Autodesk Inventor part; units mm, degrees
ref_plane "YZ Plane" through (0, 0, 0) normal (1, 0, 0) x (0, 1, 0)
ref_plane "XZ Plane" through (0, 0, 0) normal (0, 1, 0) x (-1, 0, 0)
ref_plane "XY Plane" through (0, 0, 0) normal (0, 0, 1) x (1, 0, 0)
sketch "Sketch1" plane through (0, 0, 0) normal (0, 0, 1) x (1, 0, 0)
  line L0 (0, 0) -> (20, 0)
  line L1 (20, 0) -> (20, 25)
  line L2 (20, 25) -> (0, 25)
  line L3 (0, 25) -> (0, 0)
  line L4 (5, 16.5) -> (17, 16.5)
  line L5 (17, 16.5) -> (17, 8.5)
  line L6 (17, 8.5) -> (5, 8.5)
  line L7 (5, 8.5) -> (5, 16.5)
  point P0 (17, 12.5)
  point P1 (20, 12.5)
  dimension "d0" = 20
  dimension "d2" = 25
  dimension "d3" = 8
  dimension "d4" = 12
  dimension "d5" = 3
extrude "Extrusion1" add sketch "Sketch1" along normal blind 3
sketch "Sketch2" plane through (0, 0, 3) normal (0, 0, 1) x (1, 0, 0)
  line L0 (17, 16.5) -> (17, 8.5)
  line L1 (17, 8.5) -> (5, 8.5)
  line L2 (5, 8.5) -> (5, 16.5)
  line L3 (5, 16.5) -> (17, 16.5)
  line L4 (20, 0) -> (20, 25)
  line L5 (20, 19.5) -> (20, 5.5)
  line L6 (20, 5.5) -> (2, 5.5)
  line L7 (2, 5.5) -> (2, 19.5)
  line L8 (2, 19.5) -> (20, 19.5)
extrude "Extrusion2" add sketch "Sketch2" along normal blind 7
sketch "Sketch3" plane through (0, 0, 10) normal (0, 0, 1) x (1, 0, 0)
  line L0 (17, 8.5) -> (5, 8.5)
  line L1 (5, 8.5) -> (5, 16.5)
  line L2 (5, 16.5) -> (17, 16.5)
  line L3 (17, 16.5) -> (17, 8.5)
  point P0 (0, 0)
extrude "Extrusion3" add sketch "Sketch3" against normal blind 3
sketch "Sketch4" plane through (0, 0, 0) normal (0, 0, -1) x (-1, 0, 0)
  line L0 (0, 0) -> (-20, 0)
  line L1 (-20, 25) -> (0, 25)
  line L2 (-20, 0) -> (-20, 25)
  circle A0 centre (-16.75, 22) radius 1.25
  circle A1 centre (-12.25, 22) radius 1.25
  circle A2 centre (-7.75, 22) radius 1.25
  circle A3 centre (-3.25, 22) radius 1.25
  circle A4 centre (-16.75, 3) radius 1.25
  circle A5 centre (-12.25, 3) radius 1.25
  circle A6 centre (-7.75, 3) radius 1.25
  circle A7 centre (-3.25, 3) radius 1.25
  line L3 (-12.25, 22) -> (-7.75, 22)
  line L4 (-17, 8.5) -> (-17, 16.5)
  line L5 (-17, 16.5) -> (-5, 16.5)
  circle A8 centre (-9, 12.5) radius 1.6
  line L6 (-5, 16.5) -> (-5, 8.5)
  point P0 (-10, 22)
  point P1 (-10, 25)
  point P2 (-17, 12.5)
  point P3 (-11, 16.5)
  dimension "d12" = 2.5
  dimension "d13" = 2.5
  dimension "d14" = 2.5
  dimension "d15" = 2.5
  dimension "d16" = 2.5
  dimension "d17" = 2.5
  dimension "d18" = 2.5
  dimension "d19" = 2.5
  dimension "d20" = 4.5
  dimension "d21" = 4.5
  dimension "d22" = 4.5
  dimension "d23" = 3
  dimension "d24" = 3
  dimension "d27" = 3.2
  dimension "d28" = 4
extrude "Extrusion4" cut sketch "Sketch4" against normal blind 10
equation "\"d21\" = d20"
equation "\"d22\" = d20"
equation "\"d24\" = d23"
properties part number "end limit holder"
Can you work these out from the model? Positions are in its coordinate system, mm. A direction names the side the tool comes from. Coordinates: 2 decimals unless noted, no trailing zeros. Loops run counter-clockwise (first coordinate to the right, second up) from the corner with the lowest first, then second, coordinate; pieces in that order, holes last.
1) Imagine slicing it at D-D on y = 12.5. List the corners of the cut face in (x, z) for me, plus the area to 3 significant figures.
2) For pin 1 (4 mm diameter, centred on x = 16.75, y = 3, fed in from -Z); pin 2 (3 mm diameter, centred on x = 7.75, y = 22, fed in from +Z); pin 3 (2 mm diameter, centred on x = 3.25, y = 3, fed in from +Z); pin 4 (4 mm diameter, centred on x = 8.5, y = 13.5, fed in from -Z), each with a flat end and sliding along its axis, tell me the tip position at first contact or that it passes through.
3) Imagine slicing it at C-C on z = 8.5. List the corners of the cut face in (x, y) for me.
4) Imagine slicing it at A-A on y = 21.25. List the corners of the cut face in (x, z) for me.
5) Imagine slicing it at B-B on x = 12.25. List the corners of the cut face in (y, z) for me, plus the area to 3 significant figures.
6) Thinking about a two-plate mould opening in X: for faces 4 (the flat face through (2, 12, 6)), 5 (the flat face through (5, 12, 3)), 6 (the flat face through (10, 25, 1)), which applies, pulls with the +X half, pulls with the -X half, needs draft (parallel to the pull), parting line crosses it, or undercut?
7) Which directions (+Z, -Z, +X, -X, +Y, -Y) give clear straight access to the entire face, cutting with the end or side of a thin tool? Please do faces 1 (the flat face through (17, 13, 3)), 2 (the flat face through (11, 5.5, 6)), 3 (the flat face through (11, 19.5, 6)).
8) I need wall thicknesses on probe 1 along Y at (x, z) = (12.25, 1.2); probe 2 along Y at (x, z) = (10.5, 1.5); probe 3 along Y at (x, z) = (15, 6.75). Which ranges of each line are inside material? Lowest first, please.
Completed:
1. outline: (0, 0) - (5, 0) - (5, 7) - (7.4, 7) - (7.4, 10) - (2, 10) - (2, 3) - (0, 3) - close; (10.6, 7) - (17, 7) - (17, 0) - (20, 0) - (20, 10) - (10.6, 10) - close
1. area: 92.4 mm2
2. pin 1: stops at z = 0
2. pin 2: stops at z = 3
2. pin 3: passes through
2. pin 4: stops at z = 7
3. outline: (2, 5.5) - (20, 5.5) - (20, 19.5) - (2, 19.5) - close; hole circle Ø3.2 at (9, 12.5)
4. outline: (0, 0) - (2.25, 0) - (2.25, 3) - (0, 3) - close; (4.25, 0) - (6.75, 0) - (6.75, 3) - (4.25, 3) - close; (8.75, 0) - (11.25, 0) - (11.25, 3) - (8.75, 3) - close; (13.25, 0) - (15.75, 0) - (15.75, 3) - (13.25, 3) - close; (17.75, 0) - (20, 0) - (20, 3) - (17.75, 3) - close
5. outline: (0, 0) - (1.75, 0) - (1.75, 3) - (0, 3) - close; (4.25, 0) - (8.5, 0) - (8.5, 7) - (16.5, 7) - (16.5, 0) - (20.75, 0) - (20.75, 3) - (19.5, 3) - (19.5, 10) - (5.5, 10) - (5.5, 3) - (4.25, 3) - close; (23.25, 0) - (25, 0) - (25, 3) - (23.25, 3) - close
5. area: 102 mm2
6. face 4: pulls with the -X half
6. face 5: undercut
6. face 6: needs draft
7. face 1: -Z
7. face 2: +Z, +X, -X, -Y
7. face 3: +Z, +X, -X, +Y
8. probe 1: y = 0 to 1.75, 4.25 to 8.5, 16.5 to 20.75, 23.25 to 25
8. probe 2: y = 0 to 8.5, 16.5 to 25
8. probe 3: y = 5.5 to 8.5, 16.5 to 19.5
